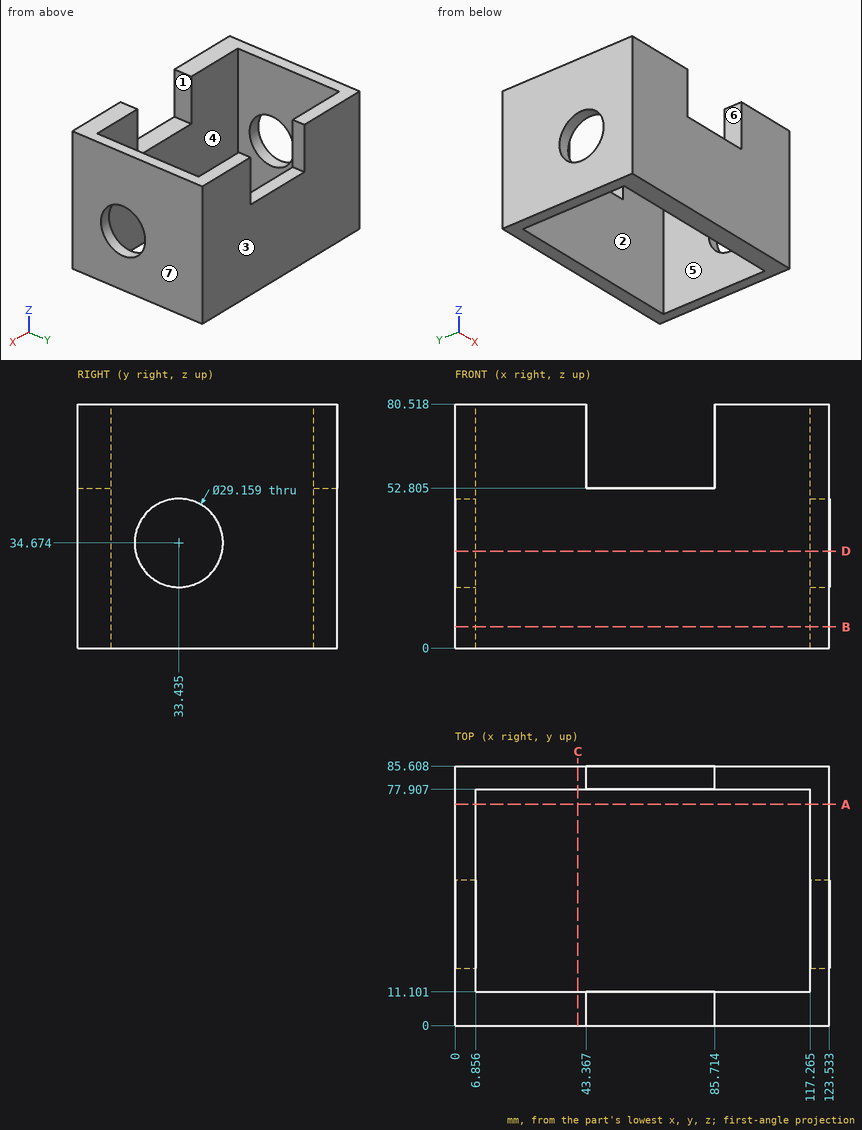
Verification items for this drawing (mm, ordinates from the low corner). A direction names the side the tool comes from. Give positions to 0.01 mm unless a question says otherwise; leave off trailing zeros. Write each loop counter-clockwise with the first axis right and the second up, starting at its lowest first coordinate (ties: lowest second). Pieces come first, ordered by that corner, then holes. Notation, with made-up numbers: (-3.75, 60) -> (16.25, 60) arc R17 cw to (16.25, 93) -> close; hole circle Ø5 at (-3.5, 62.5). An arc over 180 degrees is marked (long way). Use CSV: the item, a comma, the result in double quotes. Start each with the question number.
Q1. Tool access check on the marked faces 5, 6 and 7. Record the directions out of +Z, -Z, +X, -X, +Y, -Y that give a thin tool (end or side, any length) a straight path to the whole face; none if there is none.
Q2. Cross-section at A-A on y = 73. Enter the section's corners in (x, z) (1 decimal), and give its area (3 significant figures).
Q3. Cross-section at C-C on x = 40.5. Enter the section's corners in (y, z), and give its area (3 significant figures).
Q4. Cross-section at B-B on z = 7. Enter the section's corners in (x, y) (1 decimal).
Q5. Scan lines: line 1 along X through (y, z) = (21, 24.5) (1 decimal); line 2 along Y through (x, z) = (108, 46). Record each from-to range of solid material in increasing order.
Q6. Depth check by flat-ended pin: P1, Ø8.5, axis at x = 69, y = 83, coming from the +Z side (1 decimal). Enter the tip coordinate at first touch or a pass-through.
Q7. Release check for a two-part mould opening along Y. For the marked faces 1, 2, 3 and 4 record: +Y half, -Y half, draft (parallel to the pull), parting line (faces both ways), or undercut.
Q8. Cross-section at D-D on z = 32. Enter the section's corners in (x, y) (1 decimal), and give its area (3 significant figures).
Working result:
1,face 5,"+Z, -Z"
1,face 6,"+Z, +Y, -Y"
1,face 7,"+Z, -Z, +X, +Y, -Y"
2,outline,"(0, 0) -> (6.9, 0) -> (6.9, 80.5) -> (0, 80.5) -> close; (117.3, 0) -> (123.5, 0) -> (123.5, 80.5) -> (117.3, 80.5) -> close"
2,area,"1,060 mm^2"
3,outline,"(0, 0) -> (11.1, 0) -> (11.1, 80.52) -> (0, 80.52) -> close; (77.91, 0) -> (85.61, 0) -> (85.61, 80.52) -> (77.91, 80.52) -> close"
3,area,"1,510 mm^2"
4,outline,"(0, 0) -> (123.5, 0) -> (123.5, 85.6) -> (0, 85.6) -> close; hole (6.9, 11.1) -> (117.3, 11.1) -> (117.3, 77.9) -> (6.9, 77.9) -> close"
5,line 1,"x = 0 to 6.9, 117.3 to 123.5"
5,line 2,"y = 0 to 11.1, 77.91 to 85.61"
6,P1,"stops at z = 52.8"
7,face 1,"draft"
7,face 2,"undercut"
7,face 3,"+Y half"
7,face 4,"undercut"
8,outline,"(0, 0) -> (123.5, 0) -> (123.5, 19.1) -> (117.3, 19.1) -> (117.3, 11.1) -> (6.9, 11.1) -> (6.9, 19.1) -> (0, 19.1) -> close; (0, 47.8) -> (6.9, 47.8) -> (6.9, 77.9) -> (117.3, 77.9) -> (117.3, 47.8) -> (123.5, 47.8) -> (123.5, 85.6) -> (0, 85.6) -> close"
8,area,"2,820 mm^2"
